Check sheet for the modelled part. Datum: model origin and axes. Units: mm. A direction names the side the tool comes from. Give positions to 0.01 mm unless a question says otherwise; leave off trailing zeros. Loops run counter-clockwise (first coordinate to the right, second up) from the corner with the lowest first, then second, coordinate; pieces in that order, holes last. Notation, with made-up numbers: (80.5, -39.75) - (122.5, -39.75) arc R14 ccw to (122.5, -14.75) - close; hole circle Ø4 at (-26.5, 75). An arc over 180 degrees is marked (long way). Use CSV: the item, a comma, the result in double quotes.
from build123d import *

# Parameters (mm, degrees)
F0_R     = 73.025
F1_DEPTH = 133.35
F2_DEPTH = 25.4


with BuildPart() as f1:
    # F0 (on Front) → F1 (new body)
    with BuildSketch(Plane.XZ):
        Circle(F0_R)
        with BuildLine():
            ThreePointArc((63.2964738354, 5.08), (63.4490980572, 2.5420377112), (63.5, 0))
            ThreePointArc((63.5, 0), (63.4490980572, -2.5420377112), (63.2964738354, -5.08))
            ThreePointArc((63.2964738354, -5.08), (62.6939870382, -10.0853353566), (61.696322928, -15.0271000916))
            ThreePointArc((61.696322928, -15.0271000916), (0, -63.5), (-61.696322928, -15.0271000916))
            ThreePointArc((-61.696322928, -15.0271000916), (-62.6939870382, -10.0853353566), (-63.2964738354, -5.08))
            ThreePointArc((-63.2964738354, -5.08), (-63.5, 0), (-63.2964738354, 5.08))
            ThreePointArc((-63.2964738354, 5.08), (-62.6939870382, 10.0853353566), (-61.696322928, 15.0271000916))
            ThreePointArc((-61.696322928, 15.0271000916), (0, 63.5), (61.696322928, 15.0271000916))
            ThreePointArc((61.696322928, 15.0271000916), (62.6939870382, 10.0853353566), (63.2964738354, 5.08))
        make_face(mode=Mode.SUBTRACT)
        with BuildLine():
            ThreePointArc((63.2964738354, -5.08), (63.4490980572, -2.5420377112), (63.5, 0))
            ThreePointArc((63.5, 0), (63.4490980572, 2.5420377112), (63.2964738354, 5.08))
            Line((63.2964738354, 5.08), (50.5231209099, 5.08))
            Line((50.5231209099, 5.08), (-8.6646769196, 5.08))
            Line((-8.6646769196, 5.08), (-51.9901923835, 5.08))
            Line((-51.9901923835, 5.08), (-63.2964738354, 5.08))
            ThreePointArc((-63.2964738354, 5.08), (-63.5, 0), (-63.2964738354, -5.08))
            Line((-63.2964738354, -5.08), (-51.9901923835, -5.08))
            Line((-51.9901923835, -5.08), (-8.6646769196, -5.08))
            Line((-8.6646769196, -5.08), (50.5231209099, -5.08))
            Line((50.5231209099, -5.08), (63.2964738354, -5.08))
        make_face()
        with BuildLine():
            Line((50.5231209099, 5.08), (63.2964738354, 5.08))
            ThreePointArc((63.2964738354, 5.08), (62.6939870382, 10.0853353566), (61.696322928, 15.0271000916))
            add(Edge.make_bspline(
                [(61.696322928, 15.0271000916), (60.4599662433, 13.2835631459), (57.8112317295, 9.5482604282), (53.0577875896, 6.6339762092), (50.5231209099, 5.08)],
                knots=[0, 0, 0, 0, 0.4667725958, 1, 1, 1, 1], degree=3))
        make_face()
        with BuildLine():
            ThreePointArc((61.696322928, -15.0271000916), (62.6939870382, -10.0853353566), (63.2964738354, -5.08))
            Line((63.2964738354, -5.08), (50.5231209099, -5.08))
            add(Edge.make_bspline(
                [(61.696322928, -15.0271000916), (60.4599662433, -13.2835631459), (57.8112317295, -9.5482604282), (53.0577875896, -6.6339762092), (50.5231209099, -5.08)],
                knots=[0, 0, 0, 0, 0.4667725958, 1, 1, 1, 1], degree=3))
        make_face()
        with BuildLine():
            add(Edge.make_bspline(
                [(-61.696322928, 15.0271000916), (-61.1179777584, 13.2619750664), (-59.7584225638, 9.3012859588), (-54.7646458459, 6.5824467775), (-51.9901923835, 5.08)],
                knots=[0, 0, 0, 0, 0.4461018831, 1, 1, 1, 1], degree=3))
            ThreePointArc((-61.696322928, 15.0271000916), (-62.6939870382, 10.0853353566), (-63.2964738354, 5.08))
            Line((-63.2964738354, 5.08), (-51.9901923835, 5.08))
        make_face()
        with BuildLine():
            ThreePointArc((-63.2964738354, -5.08), (-62.6939870382, -10.0853353566), (-61.696322928, -15.0271000916))
            add(Edge.make_bspline(
                [(-61.696322928, -15.0271000916), (-61.1179777584, -13.2619750664), (-59.7584225638, -9.3012859588), (-54.7646458459, -6.5824467775), (-51.9901923835, -5.08)],
                knots=[0, 0, 0, 0, 0.4461018831, 1, 1, 1, 1], degree=3))
            Line((-51.9901923835, -5.08), (-63.2964738354, -5.08))
        make_face()
    extrude(amount=F1_DEPTH)

    # F0 (on Front) → F2 (join)
    with BuildSketch(Plane.XZ):
        with BuildLine():
            add(Edge.make_bspline(
                [(61.696322928, 15.0271000916), (60.4599662433, 13.2835631459), (57.8112317295, 9.5482604282), (53.0577875896, 6.6339762092), (50.5231209099, 5.08)],
                knots=[0, 0, 0, 0, 0.4667725958, 1, 1, 1, 1], degree=3))
            ThreePointArc((61.696322928, 15.0271000916), (0, 63.5), (-61.696322928, 15.0271000916))
            add(Edge.make_bspline(
                [(-61.696322928, 15.0271000916), (-61.1179777584, 13.2619750664), (-59.7584225638, 9.3012859588), (-54.7646458459, 6.5824467775), (-51.9901923835, 5.08)],
                knots=[0, 0, 0, 0, 0.4461018831, 1, 1, 1, 1], degree=3))
            Line((-51.9901923835, 5.08), (-8.6646769196, 5.08))
            Line((-8.6646769196, 5.08), (50.5231209099, 5.08))
        make_face()
        with BuildLine():
            ThreePointArc((-61.696322928, -15.0271000916), (0, -63.5), (61.696322928, -15.0271000916))
            add(Edge.make_bspline(
                [(61.696322928, -15.0271000916), (60.4599662433, -13.2835631459), (57.8112317295, -9.5482604282), (53.0577875896, -6.6339762092), (50.5231209099, -5.08)],
                knots=[0, 0, 0, 0, 0.4667725958, 1, 1, 1, 1], degree=3))
            Line((50.5231209099, -5.08), (-8.6646769196, -5.08))
            Line((-8.6646769196, -5.08), (-51.9901923835, -5.08))
            add(Edge.make_bspline(
                [(-61.696322928, -15.0271000916), (-61.1179777584, -13.2619750664), (-59.7584225638, -9.3012859588), (-54.7646458459, -6.5824467775), (-51.9901923835, -5.08)],
                knots=[0, 0, 0, 0, 0.4461018831, 1, 1, 1, 1], degree=3))
        make_face()
    extrude(amount=F2_DEPTH)


solid = f1.part
1. Release check for a two-part mould opening along Z. For faces 3 (the face through (69.653, -65.742, 21.935)), 4 (the face through (1, -25.4, 28)), 5 (the face through (-6, -133.35, 0)) record: released by +Z, released by -Z, zero draft, split by the parting line, or undercut.
Completed:
face 3,"split by the parting line"
face 4,"undercut"
face 5,"zero draft"
2. Sectioned sample at A-A, the plane x = 0. Record the boundary of the cut face in (y, z) (3 decimals), and give its area (3 significant figures).
Completed:
outline,"(-133.35, -73.025) - (0, -73.025) - (0, 73.025) - (-133.35, 73.025) - (-133.35, 63.5) - (-25.4, 63.5) - (-25.4, 5.08) - (-133.35, 5.08) - (-133.35, -5.08) - (-25.4, -5.08) - (-25.4, -63.5) - (-133.35, -63.5) - close"
area,"6,860 mm²"
3. Scan lines: line 1 along Z through (x, y) = (-53.5, -64.5); line 2 along Z through (x, y) = (45, -94); line 3 along X through (y, z) = (-50, -15). Record each from-to range of solid material in increasing order.
Completed:
line 1,"z = -49.7 to -34.21, -5.9 to 5.9, 34.21 to 49.7"
line 2,"z = -57.51 to -44.8, -5.08 to 5.08, 44.8 to 57.51"
line 3,"x = -71.47 to -61.69, 61.68 to 71.47"
4. Sectioned sample at B-B, the plane z = -56. Record the boundary of the cut face in (x, y).
Completed:
outline,"(-46.87, -133.35) - (-29.94, -133.35) - (-29.94, -25.4) - (29.94, -25.4) - (29.94, -133.35) - (46.87, -133.35) - (46.87, 0) - (-46.87, 0) - close"
5. Go/stop test with flat-tipped pins: pin 1 Ø10 at (x, y) = (-8, -95.5) entering from +Z; pin 2 Ø3 at (y, z) = (-101, -34.5) entering from +X; pin 3 Ø5 at (y, z) = (-21, -6) entering from +X. Record where each tip stops, or that it passes through.
Completed:
pin 1,"stops at z = 72.96"
pin 2,"stops at x = 65.14"
pin 3,"stops at x = 72.94"
6. Set-up check for faces 1 (the face through (1, 0, 1)), 2 (the face through (-1, -25.4, -27)): record each of +Z, -Z, +X, -X, +Y, -Y from which the full face is reachable in a straight line by a thin tool's end or side.
Completed:
face 1,"+Z, -Z, +X, -X, +Y"
face 2,"-Y"
7. Sectioned sample at D-D, the plane y = -19.5. Record the boundary of the cut face in (x, z) (3 decimals), and give its area (3 significant figures).
Completed:
outline,"circle Ø146.05 at (0, 0)"
area,"16,800 mm²"
8. Sectioned sample at C-C, the plane y = -44. State how many separate pieces and enclosed holes the cut face has, and give its area (3 significant figures).
Completed:
separate pieces,"1"
enclosed holes,"2"
area,"5,570 mm²"
